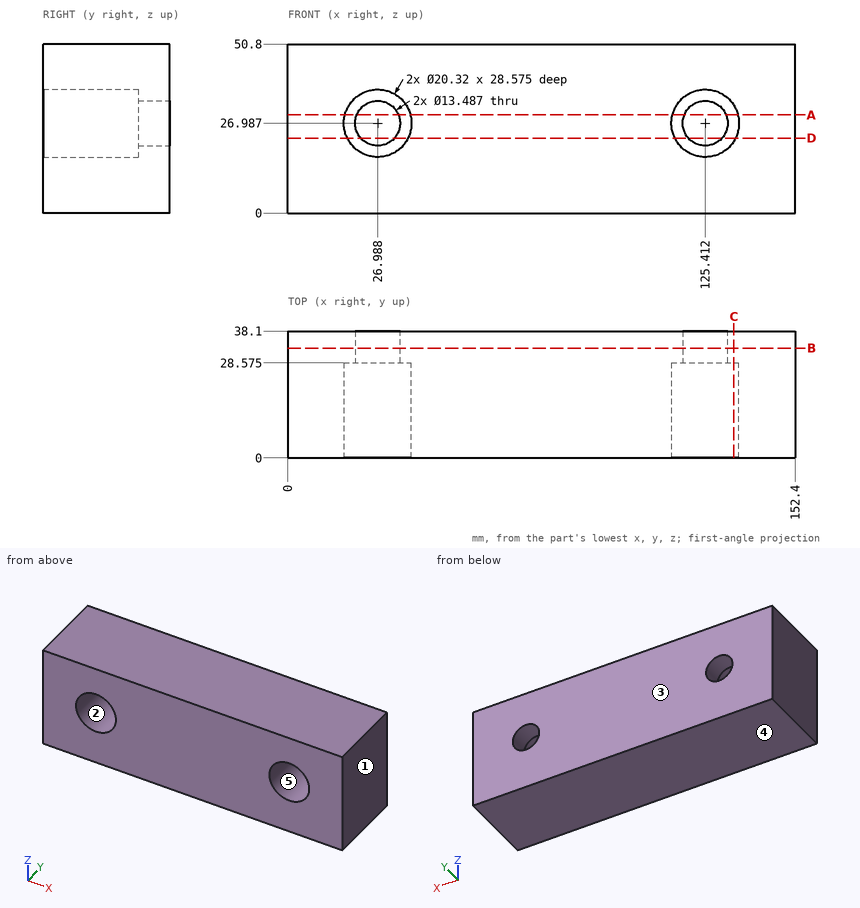
Check sheet for the drawn part. Datum: minimum x, y, z corner. Units: mm. A direction names the side the tool comes from. Round coordinates to 2 decimals unless told otherwise and drop trailing zeros. Order: outer loops, then holes, each group sorted by start corner. A loop starts at its lowest first (then second) coordinate and runs counter-clockwise, first axis right, second up. Notation, with made-up numbers: (68, -33.5) -> (74, -33.5) arc R24 ccw to (74, -1.5) -> close; hole circle Ø1 at (39, 56). An arc over 180 degrees is marked (long way). Put each result on its own line as item: value.
1) Mould release check, pull along Z, two halves, no side actions. Record for the marked faces 3, 4 and 5: +Z half, -Z half, draft (parallel to the pull), parting line (faces both ways), or undercut.
Final values:
face 3: draft
face 4: -Z half
face 5: undercut
2) Depth check by flat-ended pin: pin 1 (10 mm diameter, centred on x = 127.5, z = 23.5, fed in from -Y) (1 decimal). Enter the tip coordinate at first touch or a pass-through.
Final values:
pin 1: stops at y = 28.6
3) Material ranges on line 1 (X direction, y = 6.5, z = 22) (1 decimal); line 2 (X direction, y = 16, z = 24); line 3 (Y direction, x = 25.5, z = 37) (1 decimal), recorded low to high.
Final values:
line 1: x = 0 to 18.1, 35.8 to 116.6, 134.3 to 152.4
line 2: x = 0 to 17.28, 36.7 to 115.7, 135.12 to 152.4
line 3: y = 28.6 to 38.1
4) Section check C-C (x = 134). Record the cut outline in (y, z) (1 decimal), then the cut area to 4 significant figures.
Final values:
outline: (0, 0) -> (38.1, 0) -> (38.1, 50.8) -> (0, 50.8) -> (0, 32.4) -> (28.6, 32.4) -> (28.6, 21.6) -> (0, 21.6) -> close
area: 1,625 mm^2
5) Set-up check for the marked faces 1 and 2: record each of +Z, -Z, +X, -X, +Y, -Y from which the full face is reachable in a straight line by a thin tool's end or side.
Final values:
face 1: +Z, -Z, +X, +Y, -Y
face 2: -Y
6) Section check A-A (z = 29.5). Record the cut outline in (x, y) (1 decimal), then the cut area to 3 significant figures.
Final values:
outline: (0, 0) -> (17.1, 0) -> (17.1, 28.6) -> (20.7, 28.6) -> (20.7, 38.1) -> (0, 38.1) -> close; (33.2, 28.6) -> (36.8, 28.6) -> (36.8, 0) -> (115.6, 0) -> (115.6, 28.6) -> (119.2, 28.6) -> (119.2, 38.1) -> (33.2, 38.1) -> close; (131.7, 28.6) -> (135.3, 28.6) -> (135.3, 0) -> (152.4, 0) -> (152.4, 38.1) -> (131.7, 38.1) -> close
area: 4,440 mm^2
7) Section check B-B (y = 33). Record the cut outline in (x, z).
Final values:
outline: (0, 0) -> (152.4, 0) -> (152.4, 50.8) -> (0, 50.8) -> close; hole circle Ø13.49 at (26.99, 26.99); hole circle Ø13.49 at (125.41, 26.99)
8) Section check D-D (z = 22.5). Record the cut outline in (x, y) (1 decimal), then the cut area to 3 significant figures.
Final values:
outline: (0, 0) -> (17.9, 0) -> (17.9, 28.6) -> (22, 28.6) -> (22, 38.1) -> (0, 38.1) -> close; (32, 28.6) -> (36.1, 28.6) -> (36.1, 0) -> (116.3, 0) -> (116.3, 28.6) -> (120.4, 28.6) -> (120.4, 38.1) -> (32, 38.1) -> close; (130.4, 28.6) -> (134.5, 28.6) -> (134.5, 0) -> (152.4, 0) -> (152.4, 38.1) -> (130.4, 38.1) -> close
area: 4,570 mm^2
